Source: CAD feature listing. Evaluate the final solid. Frame: model axes, mm. A direction names the side the tool comes from. Give positions to 0.01 mm unless a question says otherwise; leave off trailing zeros. Loops run counter-clockwise (first coordinate to the right, second up) from the corner with the lowest first, then second, coordinate; pieces in that order, holes last. Notation, with made-up numbers: (6, 38.5) -> (62, 38.5) arc R15 ccw to (62, 51.5) -> close; hole circle Ø10 at (58.25, -19.5). An arc over 180 degrees is marked (long way). Answer as a JSON object with one key per item and string values. Group by question number.
from build123d import *

# Parameters (mm, degrees)
F1_DEPTH  = 617.22
F0_W      = 19.05
F0_H      = 127
F2_DEPTH  = 596.9
F3_DEPTH  = 152.4
F6_ANGLE  = 90
F12_ANGLE = -90
F18_ANGLE = 90
F19_ANGLE = 90
F23_ANGLE = 90
F24_ANGLE = 90
F25_DEPTH = 5.08
F26_DEPTH = 5.08
F27_R     = 12.7


with BuildPart() as f1:
    # F0 (on Front) → F1 (new body)
    with BuildSketch(Plane.XZ):
        with BuildLine():
            Line((19.05, 127), (19.05, 63.5))
            Line((19.05, 63.5), (82.55, 63.5))
            ThreePointArc((82.55, 63.5), (63.9512806053, 108.4012806053), (19.05, 127))
        make_face()
        with BuildLine():
            Line((19.05, 63.5), (19.05, 0))
            ThreePointArc((19.05, 0), (63.9512806053, 18.5987193947), (82.55, 63.5))
            Line((82.55, 63.5), (19.05, 63.5))
        make_face()
        Polygon((0, 127), (0, 0), (19.05, 0), (19.05, 63.5), (19.05, 127), align=None)
    extrude(amount=F1_DEPTH)


with BuildPart() as f2:
    # F0 (on Front) → F2 (new body)
    with BuildSketch(Plane.XZ):
        with Locations((249.8001466751, 63.5)):
            Rectangle(F0_W, F0_H)
        with BuildLine():
            ThreePointArc((240.2751466751, 127), (195.3738660698, 108.4012806053), (176.7751466751, 63.5))
            ThreePointArc((176.7751466751, 63.5), (195.3738660698, 18.5987193947), (240.2751466751, 0))
            Line((240.2751466751, 0), (240.2751466751, 127))
        make_face()
    extrude(amount=F2_DEPTH)


with BuildPart() as f3:
    # F0 (on Front) → F3 (new body)
    with BuildSketch(Plane.XZ):
        with BuildLine():
            ThreePointArc((-240.2751466751, 0), (-195.3738660698, 18.5987193947), (-176.7751466751, 63.5))
            ThreePointArc((-176.7751466751, 63.5), (-195.3738660698, 108.4012806053), (-240.2751466751, 127))
            Line((-240.2751466751, 127), (-240.2751466751, 0))
        make_face()
        with Locations((-249.8001466751, 63.5)):
            Rectangle(F0_W, F0_H)
    extrude(amount=F3_DEPTH)


with BuildPart() as f4_1:
    # F4: copy of F3
    add(f3.part.moved(Location((127, 0, 0))))


with BuildPart() as f5_1:
    # F5: copy of F1
    add(f1.part.moved(Location((127, 127, 254))))


with BuildPart() as f5_1_1:
    # F6: moved
    add(f5_1.part.rotate(Axis((127, 127, 317.5), (0, 0, 1)), F6_ANGLE))


with BuildPart() as f5_1_2:
    # F9: moved
    add(f5_1_1.part.moved(Location((0, -127, -254))))


with BuildPart() as f5_1_3:
    # F11: moved
    add(f5_1_2.part.moved(Location((132.3251466751, 0, 0))))


with BuildPart() as f1_1:
    # F12: moved
    add(f1.part.rotate(Axis((0, -617.22, 63.5), (0, 0, 1)), F12_ANGLE))


with BuildPart() as f1_2:
    # F14: moved
    add(f1_1.part.moved(Location((0, 20.32, 0))))


with BuildPart() as f1_3:
    # F16: moved
    add(f1_2.part.moved(Location((259.3251466751, 0, 0))))


    add(f2.part)  # F18 merges F2
    # F2_face1 (on face) → F18 (revolve)
    with BuildSketch(Plane(origin=(223.4065289788, -596.9, 63.5), x_dir=(1, 0, 0), z_dir=(0, -1, 0))):
        with BuildLine():
            Line((35.9186176963, 63.5), (16.8686176963, 63.5))
            ThreePointArc((16.8686176963, 63.5), (-46.6313823037, 0), (16.8686176963, -63.5))
            Line((16.8686176963, -63.5), (35.9186176963, -63.5))
            Line((35.9186176963, -63.5), (35.9186176963, 63.5))
        make_face()
    revolve(axis=Axis((259.3251466751, -596.9, 63.5), (0, 0, 1)), revolution_arc=F18_ANGLE)


    add(f5_1_3.part)  # F19 merges F5_1
    # F0 (on Front) → F19 (revolve)
    with BuildSketch(Plane.XZ):
        with Locations((249.8001466751, 63.5)):
            Rectangle(F0_W, F0_H)
        with BuildLine():
            ThreePointArc((240.2751466751, 127), (195.3738660698, 108.4012806053), (176.7751466751, 63.5))
            ThreePointArc((176.7751466751, 63.5), (195.3738660698, 18.5987193947), (240.2751466751, 0))
            Line((240.2751466751, 0), (240.2751466751, 127))
        make_face()
    revolve(axis=Axis((259.3251466751, 0, 63.5), (0, 0, -1)), revolution_arc=F19_ANGLE)



with BuildPart() as f4_1_1:
    # F21: moved
    add(f4_1.part.moved(Location((1008.8702933502, -444.5, 0))))


with BuildPart() as f3_1:
    # F22: moved
    add(f3.part.moved(Location((1135.8702933502, 0, 0))))


with BuildPart() as f1_4:
    add(f1_3.part)

    add(f3_1.part)  # F23 merges F3
    # F5_face1 (on face) → F23 (revolve)
    with BuildSketch(Plane(origin=(876.5451466751, 35.9186176963, 63.5), x_dir=(0, 1, 0), z_dir=(1, 0, 0))):
        with BuildLine():
            ThreePointArc((-16.8686176963, -63.5), (46.6313823037, 0), (-16.8686176963, 63.5))
            Line((-16.8686176963, 63.5), (-35.9186176963, 63.5))
            Line((-35.9186176963, 63.5), (-35.9186176963, -63.5))
            Line((-35.9186176963, -63.5), (-16.8686176963, -63.5))
        make_face()
    revolve(axis=Axis((876.5451466751, 0, 63.5), (0, 0, -1)), revolution_arc=F23_ANGLE)


    add(f4_1_1.part)  # F24 merges F4_1
    # F1_face2 (on face) → F24 (revolve)
    with BuildSketch(Plane(origin=(876.5451466751, -632.8186176963, 63.5), x_dir=(0, 1, 0), z_dir=(1, 0, 0))):
        with BuildLine():
            ThreePointArc((16.8686176963, 63.5), (-46.6313823037, 0), (16.8686176963, -63.5))
            Line((16.8686176963, -63.5), (35.9186176963, -63.5))
            Line((35.9186176963, -63.5), (35.9186176963, 63.5))
            Line((35.9186176963, 63.5), (16.8686176963, 63.5))
        make_face()
    revolve(axis=Axis((876.5451466751, -596.9, 63.5), (0, 0, 1)), revolution_arc=F24_ANGLE)

    # F25 (add): a face of the model
    f25_faces = [f1_4.faces().sort_by_distance(p)[0] for p in [
        (912.4637643715, -444.5, 63.5),
    ]]
    extrude(f25_faces, amount=F25_DEPTH)

    # F26 (add): a face of the model
    f26_faces = [f1_4.faces().sort_by_distance(p)[0] for p in [
        (912.4637643715, -152.4, 63.5),
    ]]
    extrude(f26_faces, amount=F26_DEPTH)

    # F27
    f27_edges = [f1_4.edges().sort_by_distance(p)[0] for p in [
        (959.095147, -439.42, 63.5),
        (886.070147, -439.42, 127),
        (886.070147, -439.42, 0),
        (959.095147, -157.48, 63.5),
        (886.070147, -157.48, 127),
        (886.070147, -157.48, 0),
    ]]
    fillet(f27_edges, radius=F27_R)


solid = f1_4.part
(1) Section query C-C on y = -196.5. Return the cut outline in (x, z).
(2) Material intervals for line 1 (Y direction, x = 409, z = 61); line 2 (X direction, y = -540.5, z = 63); line 3 (Y direction, x = 331, z = 58.5), sorted ascending. Write a range as from..to.
(3) Section query B-B on y = -561. Return the cut outline in (x, z), plus the area to 3 significant figures.
(4) Section query A-A on x = 821. Return the cut outline in (y, z), plus the area to 3 significant figures.
(5) Access query for faces 4 (the face through (876.545, -519, 63)), 5 (the face through (959.08, -71.38, 62.1)), 6 (the face through (903, -439.42, 64)). Directions: +Z, -Z, +X, -X, +Y, -Y. A direction counts if a zero-diameter tool reaches every point of the face in a straight line with its end or side. Return the directions, or none.
(6) First-contact query: pin 1 (2 mm diameter, centred on x = 618, z = 34.5, fed in from -Y); pin 2 (10 mm diameter, centred on x = 522, z = 27.5, fed in from +Y); pin 3 (2 mm diameter, centred on y = -367.5, z = 29.5, fed in from -X). Flat tips, straight axial feed; report the tip coordinate or a pass-through.
(7) Mould query, pull axis X, two halves, no side actions, for faces 1 (the face through (903, -157.48, 64)), 2 (the face through (564, 0, 64)), 3 (the face through (959.08, -525.52, 62.1)). Classes: pulls with the +X half, pulls with the -X half, needs draft (parallel to the pull), parting line crosses it, or undercut.
Result:
{
 "1": {"outline": "(240.28, 0) -> (259.33, 0) -> (259.33, 127) -> (240.28, 127) arc R63.5 ccw to start"},
 "2": {"line 1": "-679.4..-596.9, 0..82.5", "line 2": "176.78..259.33, 876.55..959.09", "line 3": "-679.25..-596.9, 0..82.35"},
 "3": {"outline": "(240.28, 0) -> (259.33, 0) -> (259.33, 127) -> (240.28, 127) arc R63.5 ccw to start; (876.55, 0) -> (895.6, 0) arc R63.5 ccw to (895.6, 127) -> (876.55, 127) -> close", "area": "17,500 mm²"},
 "4": {"outline": "(-615.95, 0) -> (-596.9, 0) -> (-596.9, 127) -> (-615.95, 127) arc R63.5 ccw to start; (0, 0) -> (19.05, 0) arc R63.5 ccw to (19.05, 127) -> (0, 127) -> close", "area": "17,500 mm²"},
 "5": {"face 4": "+Z, -Z", "face 5": "+X, +Y, -Y", "face 6": "+Z, -Z, +X"},
 "6": {"pin 1": "y = -672.94", "pin 2": "y = 74.47", "pin 3": "x = 186.02"},
 "7": {"face 1": "needs draft", "face 2": "undercut", "face 3": "pulls with the +X half"}
}
